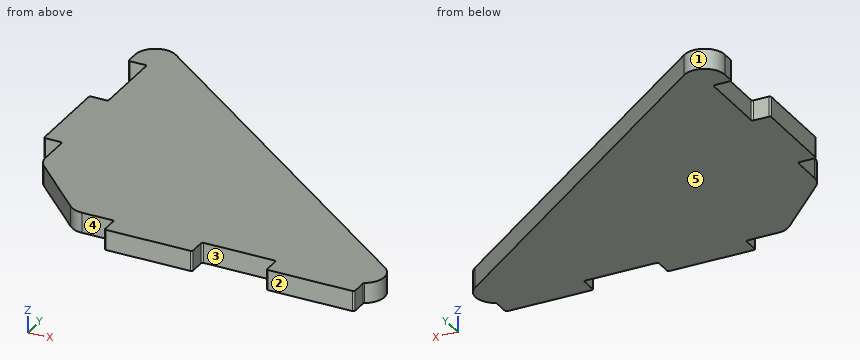
from build123d import *

# Parameters (mm, degrees)
BASE_FLANGE1_DEPTH = 4.7625
FILLET1_R          = 0.396875
FILLET2_R          = 4.7625


# Sheet-metal steps are written as plain solids
with BuildPart() as part:
    # Sketch1 → Base-Flange1 (new body)
    with BuildSketch(Plane.XY):
        Polygon((-4.365625, 76.2), (95.25, 0), (84.1375, 0), (84.1375, -4.365625), (63.5, -4.365625), (63.5, 0), (46.0375, 0), (46.0375, -4.365625), (25.4, -4.365625), (25.4, 0), (15.875, 0), (0, 15.875), (0, 25.4), (-4.365625, 25.4), (-4.365625, 46.0375), (0, 46.0375), (0, 63.5), (-4.365625, 63.5), align=None)
    extrude(amount=-BASE_FLANGE1_DEPTH)

    # Fillet1
    fillet1_edges = [part.edges().sort_by_distance(p)[0] for p in [
        (25.4, 0, -2.38125),
        (0, 25.4, -2.38125),
        (-4.365625, 25.4, -2.38125),
        (-4.365625, 46.0375, -2.38125),
        (0, 46.0375, -2.38125),
        (0, 63.5, -2.38125),
        (-4.365625, 63.5, -2.38125),
        (84.1375, 0, -2.38125),
        (84.1375, -4.365625, -2.38125),
        (63.5, -4.365625, -2.38125),
        (63.5, 0, -2.38125),
        (46.0375, 0, -2.38125),
        (46.0375, -4.365625, -2.38125),
        (25.4, -4.365625, -2.38125),
    ]]
    fillet(fillet1_edges, radius=FILLET1_R)

    # Fillet2
    fillet2_edges = [part.edges().sort_by_distance(p)[0] for p in [
        (95.25, 0, -2.38125),
        (15.875, 0, -2.38125),
        (0, 15.875, -2.38125),
        (-4.365625, 76.2, -2.38125),
    ]]
    fillet(fillet2_edges, radius=FILLET2_R)


solid = part.part
Can you work these out from the model? Positions are in its coordinate system, mm. Face numbers are marked on the shaded views. A direction names the side the tool comes from. Round coordinates to 2 decimals unless told otherwise and drop trailing zeros. Order: outer loops, then holes, each group sorted by start corner. A loop starts at its lowest first (then second) coordinate and runs counter-clockwise, first axis right, second up. Notation, with made-up numbers: (-17, -21.75) - (19, -21.75) arc R37 cw to (19, 17.25) - close; hole circle Ø7 at (35, -35). An arc over 180 degrees is marked (long way). Answer in a Markdown table with one row per item.
(1) Suppose I cut it at B-B, the plane x = 54. Please give me the cut outline in (y, z).
From the geometry:
| item | result |
|---|---|
| outline | (0, -4.76) - (31.55, -4.76) - (31.55, 0) - (0, 0) - close |
(2) Please list where these lines run through material, in increasing order: L1, parallel to Y at x = 45, z = -0.65; L2, parallel to Y at x = 57, z = -1.1; L3, parallel to X at y = 34.5, z = -3.25. Write a range as from..to.
From the geometry:
| item | result |
|---|---|
| L1 | y = -4.37..38.44 |
| L2 | y = 0..29.26 |
| L3 | x = -4.37..50.15 |
(3) Which directions (+Z, -Z, +X, -X, +Y, -Y) give clear straight access to the entire face, cutting with the end or side of a thin tool? Please do the marked faces 4 and 5.
From the geometry:
| item | result |
|---|---|
| face 4 | +Z, -Z, -X, -Y |
| face 5 | -Z, +X, -X, +Y, -Y |
(4) If we mould it in two halves opening along X, with no side actions, what happens to the marked faces 1, 2 and 3? For each: released by +X, released by -X, zero draft, split by the parting line, or undercut.
From the geometry:
| item | result |
|---|---|
| face 1 | split by the parting line |
| face 2 | zero draft |
| face 3 | undercut |
(5) Suppose I cut it at A-A, the plane y = 61.5. Please give me the cut outline in (x, z).
From the geometry:
| item | result |
|---|---|
| outline | (0, -4.76) - (14.85, -4.76) - (14.85, 0) - (0, 0) - close |
(6) For P1, Ø1.1, axis at y = -1.5, z = -1.5, coming from the -X side; P2, Ø1.1, axis at y = -3, z = -2, coming from the +X side; P3, Ø1.8, axis at x = -2.5, z = -1.5, coming from the +Y side, each with a flat end and sliding along its axis, tell me the tip position at first contact or that it passes through.
From the geometry:
| item | result |
|---|---|
| P1 | stops at x = 25.4 |
| P2 | stops at x = 84.14 |
| P3 | stops at y = 70.88 |
